Could you check a few things on this model? Use its own coordinates, in mm. Face numbers are marked on the shaded views. A direction names the side the tool comes from. Round coordinates to 2 decimals unless told otherwise and drop trailing zeros. Loops run counter-clockwise (first coordinate to the right, second up) from the corner with the lowest first, then second, coordinate; pieces in that order, holes last. Notation, with made-up numbers: (29, -31.75) -> (60, -31.75) arc R33 ccw to (60, 7.25) -> close; hole circle Ø2 at (15.25, 28.5). An arc over 180 degrees is marked (long way). Put each result on its own line as item: value. Start each with the question number.
1. Imagine slicing it at B-B, the plane z = 0. Please give me the cut outline in (x, y), and give its area (3 significant figures).
2. I need wall thicknesses on line 1 (Z direction, x = 3.5, y = -2.35); line 2 (X direction, y = -1.7, z = 0); line 3 (Z direction, x = -5.75, y = -1.4). Which ranges of each line are inside material? Lowest first, please. Write a range as [from, to].
3. Which directions (+Z, -Z, +X, -X, +Y, -Y) give clear straight access to the entire face, cutting with the end or side of a thin tool? Please do the marked faces 1, 2 and 3.
4. Imagine slicing it at D-D, the plane x = -10. Please give me the cut outline in (y, z), and give its area (3 significant figures).
5. If we mould it in two halves opening along Z, with no side actions, what happens to the marked faces 4, 5 and 6? For each: pulls with the +Z half, pulls with the -Z half, needs draft (parallel to the pull), parting line crosses it, or undercut.
6. Imagine slicing it at C-C, the plane y = -2.7. Please give me the cut outline in (x, z), and give its area (3 significant figures).
7. Imagine slicing it at A-A, the plane x = 3. Please give me the cut outline in (y, z).
```python
from build123d import *

# Parameters (mm, degrees)
F1_DEPTH = 3
F2_W     = 12.5
F2_H     = 13
F3_DEPTH = 1
F4_W     = 12.5
F4_H     = 13
F5_DEPTH = 1
F6_W     = 3.383816
F6_H     = 15
F7_DEPTH = 25


with BuildPart() as f1:
    # F0 (on Front) → F1 (new body)
    with BuildSketch(Plane.XZ):
        Polygon((9.25, -7.5), (9.25, 7.5), (-13.75, 7.5), (-19.133816, 7.5), (-19.133816, -7.5), (-13.75, -7.5), align=None)
        with BuildLine():
            Line((-6.25, 4.5), (6.25, 4.5))
            Line((6.25, 4.5), (6.25, -4.5))
            Line((6.25, -4.5), (-6.25, -4.5))
            ThreePointArc((-6.25, -4.5), (-10.75, 0), (-6.25, 4.5))
        make_face(mode=Mode.SUBTRACT)
    extrude(amount=F1_DEPTH)

    # F2 (on face) → F3 (cut)
    with BuildSketch(Plane.XZ.offset(3)):
        Rectangle(F2_W, F2_H)
        with BuildLine():
            Line((-6.25, -6.5), (-6.25, 6.5))
            ThreePointArc((-6.25, 6.5), (-12.75, 0), (-6.25, -6.5))
        make_face()
    extrude(amount=-F3_DEPTH, mode=Mode.SUBTRACT)

    # F4 (on face) → F5 (cut)
    with BuildSketch(Plane(origin=(0, 0, 0), x_dir=(-1, 0, 0), z_dir=(0, 1, 0))):
        Rectangle(F4_W, F4_H)
        with BuildLine():
            ThreePointArc((6.25, -6.5), (12.75, 0), (6.25, 6.5))
            Line((6.25, 6.5), (6.25, -6.5))
        make_face()
    extrude(amount=-F5_DEPTH, mode=Mode.SUBTRACT)

    # F6 (on face) → F7 (cut)
    with BuildSketch(Plane.XZ.offset(3)):
        with Locations((-17.441908, 0)):
            Rectangle(F6_W, F6_H)
    extrude(amount=-F7_DEPTH, mode=Mode.SUBTRACT)


solid = f1.part
```
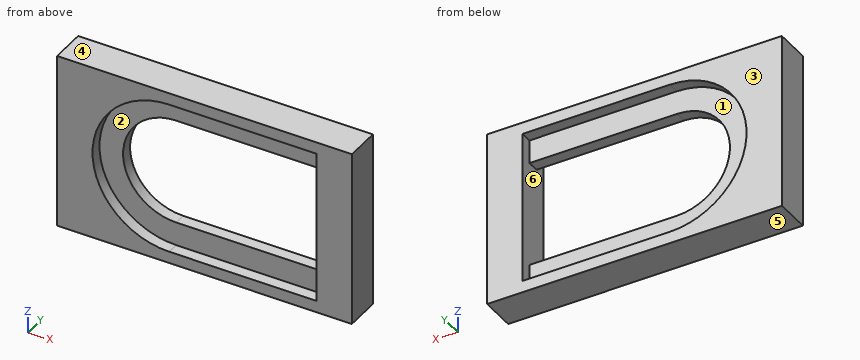
Entries:
1. outline: (-15.75, -3) -> (-12.75, -3) -> (-12.75, -2) -> (-10.75, -2) -> (-10.75, -1) -> (-12.75, -1) -> (-12.75, 0) -> (-15.75, 0) -> close; (6.25, -3) -> (9.25, -3) -> (9.25, 0) -> (6.25, 0) -> close
1. area: 20.0 mm^2
2. line 1: [-7.5, -6.5], [6.5, 7.5]
2. line 2: [-15.75, -10.75], [6.25, 9.25]
2. line 3: [-7.5, -4.5], [4.5, 7.5]
3. face 1: +Y
3. face 2: -Y
3. face 3: +Z, -Z, +X, -X, +Y
4. outline: (-3, -7.5) -> (0, -7.5) -> (0, -5.31) -> (-1, -5.31) -> (-1, -2.49) -> (-2, -2.49) -> (-2, -5.31) -> (-3, -5.31) -> close; (-3, 5.31) -> (-2, 5.31) -> (-2, 2.49) -> (-1, 2.49) -> (-1, 5.31) -> (0, 5.31) -> (0, 7.5) -> (-3, 7.5) -> close
4. area: 18.8 mm^2
5. face 4: pulls with the +Z half
5. face 5: pulls with the -Z half
5. face 6: undercut
6. outline: (-15.75, -7.5) -> (9.25, -7.5) -> (9.25, 7.5) -> (-15.75, 7.5) -> close; hole (-6.25, -6.5) -> (6.25, -6.5) -> (6.25, 6.5) -> (-6.25, 6.5) arc R6.5 ccw to start
6. area: 146 mm^2
7. outline: (-3, -7.5) -> (0, -7.5) -> (0, -6.5) -> (-1, -6.5) -> (-1, -4.5) -> (-2, -4.5) -> (-2, -6.5) -> (-3, -6.5) -> close; (-3, 6.5) -> (-2, 6.5) -> (-2, 4.5) -> (-1, 4.5) -> (-1, 6.5) -> (0, 6.5) -> (0, 7.5) -> (-3, 7.5) -> close
